from build123d import *

# Parameters (mm, degrees)
ESQUISSE1_R        = 1.5
BOSS_EXTRU_2_DEPTH = 3


with BuildPart() as part:
    # Esquisse1 → Boss.-Extru.2 (new body)
    with BuildSketch(Plane.XY):
        with BuildLine():
            Line((-5.230618988, 6.875), (-7.5, 6.875))
            Line((-7.5, 6.875), (-7.5, 8.275))
            Line((-7.5, 8.275), (7.5, 8.275))
            Line((7.5, 8.275), (7.5, 6.875))
            Line((7.5, 6.875), (5.230618988, 6.875))
            Line((5.230618988, 6.875), (5.230618988, 5.375))
            ThreePointArc((5.230618988, 5.375), (5.918936429, 4.606103727), (6.495190528, 3.75))
            ThreePointArc((6.495190528, 3.75), (10.934773091, 2.560417438), (12.124355653, 7))
            ThreePointArc((12.124355653, 7), (9.414650572, 10.36167721), (5.80943088, 12.737759334))
            ThreePointArc((5.80943088, 12.737759334), (3.975330286, 12.779130538), (2.411034891, 11.820685714))
            ThreePointArc((2.411034891, 11.820685714), (0, 10.75), (-2.411034891, 11.820685714))
            ThreePointArc((-2.411034891, 11.820685714), (-4.47014813, 12.872261577), (-6.707371512, 12.288660114))
            ThreePointArc((-6.707371512, 12.288660114), (-9.780131311, 10.017436376), (-12.124355653, 7))
            ThreePointArc((-12.124355653, 7), (-10.934773091, 2.560417438), (-6.495190528, 3.75))
            ThreePointArc((-6.495190528, 3.75), (-5.918936429, 4.606103727), (-5.230618988, 5.375))
            Line((-5.230618988, 5.375), (-5.230618988, 6.875))
        make_face()
        with Locations((9.309773091, 5.375)):
            Circle(ESQUISSE1_R, mode=Mode.SUBTRACT)
        with Locations((-9.309773091, 5.375)):
            Circle(ESQUISSE1_R, mode=Mode.SUBTRACT)
    extrude(amount=BOSS_EXTRU_2_DEPTH)


solid = part.part
Here's how the part is built. I have some questions about the finished solid (model axes, mm). A direction names the side the tool comes from. Coordinates: 2 decimals unless noted, no trailing zeros. Order: outer loops, then holes, each group sorted by start corner. A loop starts at its lowest first (then second) coordinate and runs counter-clockwise, first axis right, second up.
Item 1: For P1, Ø1, axis at y = 9, z = 2, coming from the -X side; P2, Ø1.6, axis at y = 6.5, z = 1, coming from the +X side; P3, Ø1.5, axis at y = 11, z = 2.5, coming from the +X side, each with a flat end and sliding along its axis, tell me the tip position at first contact or that it passes through.
Result sheet:
P1: stops at x = -11.12
P2: stops at x = 12.54
P3: stops at x = 9.54
Item 2: If we section it at B-B on x = 10.5: List the corners of the cut face in (y, z) for me, plus the area to 3 significant figures.
Result sheet:
outline: (2.35, 0) - (4.46, 0) - (4.46, 3) - (2.35, 3) - close; (6.29, 0) - (9.26, 0) - (9.26, 3) - (6.29, 3) - close
area: 15.3 mm2
Item 3: If we section it at D-D on y = 6: List the corners of the cut face in (x, z) for me.
Result sheet:
outline: (-12.5, 0) - (-10.67, 0) - (-10.67, 3) - (-12.5, 3) - close; (-7.95, 0) - (-5.23, 0) - (-5.23, 3) - (-7.95, 3) - close; (5.23, 0) - (7.95, 0) - (7.95, 3) - (5.23, 3) - close; (10.67, 0) - (12.5, 0) - (12.5, 3) - (10.67, 3) - close
Item 4: For faces 1 (the face through (7.5, 8, 1)), 2 (the face through (-5.93, 4.59, 1.48)), 3 (the face through (0, 9, 3)), which set-ups out of +Z, -Z, +X, -X, +Y, -Y let a thin tool reach every point of the face, with its end or its side?
Result sheet:
face 1: +Z, -Z
face 2: +Z, -Z, -Y
face 3: +Z, +X, -X, +Y, -Y
Item 5: If we section it at A-A on z = 2.05: List the corners of the cut face in (x, y) for me (3 decimals), plus the area to 3 significant figures.
Result sheet:
outline: (-12.124, 7) arc R3.25 ccw to (-6.495, 3.75) arc R7.5 cw to (-5.231, 5.375) - (-5.231, 6.875) - (-7.5, 6.875) - (-7.5, 8.275) - (7.5, 8.275) - (7.5, 6.875) - (5.231, 6.875) - (5.231, 5.375) arc R7.5 cw to (6.495, 3.75) arc R3.25 ccw to (12.124, 7) arc R14 ccw to (5.809, 12.738) arc R3.25 ccw to (2.411, 11.821) arc R3.25 cw to (-2.411, 11.821) arc R3.25 ccw to (-6.707, 12.289) arc R14 ccw to start; hole circle Ø3 at (-9.31, 5.375); hole circle Ø3 at (9.31, 5.375)
area: 126 mm2
Item 6: If we mould it in two halves opening along X, with no side actions, what happens to faces 4 (the face through (9.46, 10.32, 1.48)), 5 (the face through (-6, 6.875, 1)), 6 (the face through (0, 9, 0))? For each: +X half, -X half, draft (parallel to the pull), parting line (faces both ways), or undercut.
Result sheet:
face 4: +X half
face 5: undercut
face 6: draft
Item 7: If we section it at C-C on y = 3: List the corners of the cut face in (x, z) for me, plus the area to 3 significant figures.
Result sheet:
outline: (-11.53, 0) - (-7.09, 0) - (-7.09, 3) - (-11.53, 3) - close; (7.09, 0) - (11.53, 0) - (11.53, 3) - (7.09, 3) - close
area: 26.6 mm2
Item 8: I need wall thicknesses on line 1 (X direction, y = 6.5, z = 1.9); line 2 (X direction, y = 4.25, z = 1.6); line 3 (X direction, y = 8, z = 1.2). Which ranges of each line are inside material? Lowest first, please.
Result sheet:
line 1: x = -12.36 to -10.3, -8.32 to -5.23, 5.23 to 8.32, 10.3 to 12.36
line 2: x = -12.36 to -10.3, -8.32 to -6.18, 6.18 to 8.32, 10.3 to 12.36
line 3: x = -11.49 to -7.5, 7.5 to 11.49
